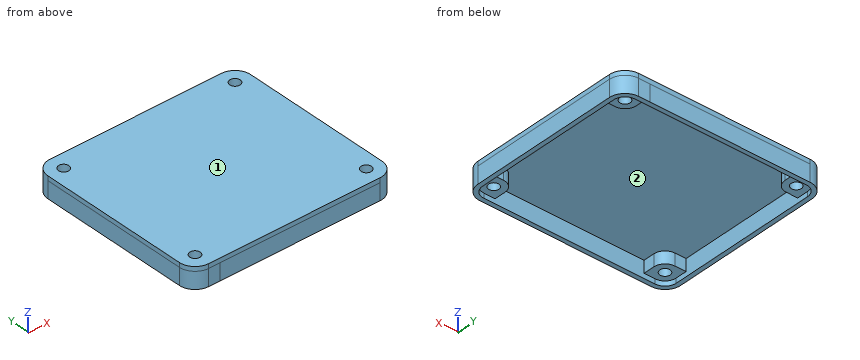
```python
from build123d import *

# Parameters (mm, degrees)
BOSS_EXTRUDE2_START     = -1.618999
SKETCH1_W               = 50.400855702
SKETCH1_H               = 1.5
SKETCH1_W_2             = 1.5
SKETCH1_H_2             = 43.400852302
BOSS_EXTRUDE2_DEPTH     = 5.668998934
SKETCH1_5_R             = 1.74999934
BOSS_EXTRUDE3_DEPTH     = 4.049997769
BOSS_EXTRUDE4_START     = 4.049997821
BOSS_EXTRUDE4_OUTLINE_R = 1.74999934
BOSS_EXTRUDE4_DEPTH     = 1.499999948


# Read off the part's stored shape, not the designer's step: Boss-Extrude4
with BuildPart() as part:
    # Sketch1 → Boss-Extrude2 (new body)
    with BuildSketch(Plane.XY.offset(BOSS_EXTRUDE2_START)):
        with BuildLine():
            Line((7.299572149, 59.8), (3.499574174, 59.8))
            ThreePointArc((3.499574174, 59.8), (-0.247791806, 58.247791067), (-1.8, 54.500424782))
            Line((-1.8, 54.500424782), (-1.8, 50.700426151))
            Line((-1.8, 50.700426151), (-0.3, 50.700426151))
            Line((-0.3, 50.700426151), (-0.3, 54.500425826))
            ThreePointArc((-0.3, 54.500425826), (0.812868735, 57.187131265), (3.499574174, 58.3))
            Line((3.499574174, 58.3), (7.299572149, 58.3))
            Line((7.299572149, 58.3), (7.299572149, 59.8))
        make_face()
        with Locations((32.5, 59.05)):
            Rectangle(SKETCH1_W, SKETCH1_H)
        with BuildLine():
            ThreePointArc((61.500425826, 59.799997355), (65.247788792, 58.247788792), (66.8, 54.500425826))
            Line((66.8, 54.500425826), (66.8, 50.700426151))
            Line((66.8, 50.700426151), (65.3, 50.700426151))
            Line((65.3, 50.700426151), (65.3, 54.500425826))
            ThreePointArc((65.3, 54.500425826), (64.18713049, 57.18713049), (61.500425826, 58.3))
            Line((61.500425826, 58.3), (57.700427851, 58.3))
            Line((57.700427851, 58.3), (57.700427851, 59.8))
            Line((57.700427851, 59.8), (61.500425826, 59.799997355))
        make_face()
        with Locations((66.05, 29)):
            Rectangle(SKETCH1_W_2, SKETCH1_H_2)
        with BuildLine():
            Line((57.700427851, -1.8), (61.500425826, -1.8))
            ThreePointArc((61.500425826, -1.8), (65.247791806, -0.247791067), (66.8, 3.499575218))
            Line((66.8, 3.499575218), (66.8, 7.299573849))
            Line((66.8, 7.299573849), (65.3, 7.299573849))
            Line((65.3, 7.299573849), (65.3, 3.499574174))
            ThreePointArc((65.3, 3.499574174), (64.187131265, 0.812868735), (61.500425826, -0.3))
            Line((61.500425826, -0.3), (57.700427851, -0.3))
            Line((57.700427851, -0.3), (57.700427851, -1.8))
        make_face()
        with Locations((32.5, -1.05)):
            Rectangle(SKETCH1_W, SKETCH1_H)
        with Locations((-1.05, 29)):
            Rectangle(SKETCH1_W_2, SKETCH1_H_2)
        with BuildLine():
            ThreePointArc((3.499576262, -1.800002645), (-0.247793343, -0.24779482), (-1.8, 3.499574174))
            Line((-1.8, 3.499574174), (-1.8, 7.299573849))
            Line((-1.8, 7.299573849), (-0.3, 7.299573849))
            Line((-0.3, 7.299573849), (-0.3, 3.499574174))
            ThreePointArc((-0.3, 3.499574174), (0.812867961, 0.812867961), (3.499574174, -0.3))
            Line((3.499574174, -0.3), (7.299572149, -0.3))
            Line((7.299572149, -0.3), (7.299572149, -1.8))
            Line((7.299572149, -1.8), (3.499576262, -1.800002645))
        make_face()
    extrude(amount=BOSS_EXTRUDE2_DEPTH)

    # Sketch1<5> → Boss-Extrude3 (add)
    # profile 1 of 4: a face of its own
    with BuildSketch(Plane.XY):
        with BuildLine():
            Line((7.299572149, 3.50000232), (7.299572149, -0.3))
            Line((7.299572149, -0.3), (3.499574174, -0.3))
            ThreePointArc((3.499574174, -0.3), (0.812867961, 0.812867961), (-0.3, 3.499574174))
            Line((-0.3, 3.499574174), (-0.3, 7.299573849))
            Line((-0.3, 7.299573849), (3.50000062, 7.299573849))
            ThreePointArc((3.50000062, 7.299573849), (6.186702813, 6.186704015), (7.299572149, 3.50000232))
        make_face()
        with Locations((3.499568884, 3.499568884)):
            Circle(SKETCH1_5_R, mode=Mode.SUBTRACT)
    # profile 2 of 4: a face of its own
    with BuildSketch(Plane.XY):
        with BuildLine():
            Line((7.299572149, 58.3), (3.499574174, 58.3))
            ThreePointArc((3.499574174, 58.3), (0.812868735, 57.187131265), (-0.3, 54.500425826))
            Line((-0.3, 54.500425826), (-0.3, 50.700426151))
            Line((-0.3, 50.700426151), (3.50000062, 50.700426151))
            ThreePointArc((3.50000062, 50.700426151), (6.186703414, 51.813294886), (7.299572149, 54.49999768))
            Line((7.299572149, 54.49999768), (7.299572149, 58.3))
        make_face()
        with Locations((3.499571529, 54.500428471)):
            Circle(SKETCH1_5_R, mode=Mode.SUBTRACT)
    # profile 3 of 4: a face of its own
    with BuildSketch(Plane.XY):
        with BuildLine():
            ThreePointArc((61.500425826, 58.3), (64.18713049, 57.18713049), (65.3, 54.500425826))
            Line((65.3, 54.500425826), (65.3, 50.700426151))
            Line((65.3, 50.700426151), (61.49999938, 50.700426151))
            ThreePointArc((61.49999938, 50.700426151), (58.813296614, 51.813295049), (57.700427851, 54.49999768))
            Line((57.700427851, 54.49999768), (57.700427851, 58.3))
            Line((57.700427851, 58.3), (61.500425826, 58.3))
        make_face()
        with Locations((61.500425826, 54.500425826)):
            Circle(SKETCH1_5_R, mode=Mode.SUBTRACT)
    # profile 4 of 4: a face of its own
    with BuildSketch(Plane.XY):
        with BuildLine():
            Line((57.700427851, -0.3), (61.500425826, -0.3))
            ThreePointArc((61.500425826, -0.3), (64.187131265, 0.812868735), (65.3, 3.499574174))
            Line((65.3, 3.499574174), (65.3, 7.299573849))
            Line((65.3, 7.299573849), (61.49999938, 7.299573849))
            ThreePointArc((61.49999938, 7.299573849), (58.813297215, 6.186703852), (57.700427851, 3.50000232))
            Line((57.700427851, 3.50000232), (57.700427851, -0.3))
        make_face()
        with Locations((61.500428471, 3.499571529)):
            Circle(SKETCH1_5_R, mode=Mode.SUBTRACT)
    extrude(amount=BOSS_EXTRUDE3_DEPTH)

    # Boss-Extrude4 outline → Boss-Extrude4 (add)
    with BuildSketch(Plane.XY.offset(BOSS_EXTRUDE4_START)):
        with BuildLine():
            ThreePointArc((-1.800001322, 3.499574174), (-0.247792408, -0.247793885), (3.499576262, -1.800001322))
            Line((3.499576262, -1.800001322), (61.500425826, -1.8))
            ThreePointArc((61.500425826, -1.8), (65.247791806, -0.247791067), (66.8, 3.499575218))
            Line((66.8, 3.499575218), (66.799998678, 54.500425826))
            ThreePointArc((66.799998678, 54.500425826), (65.247789727, 58.247789727), (61.500425826, 59.799998678))
            Line((61.500425826, 59.799998678), (3.499574174, 59.8))
            ThreePointArc((3.499574174, 59.8), (-0.247791806, 58.247791067), (-1.8, 54.500424782))
            Line((-1.8, 54.500424782), (-1.800001322, 3.499574174))
        make_face()
        with Locations((3.499568884, 3.499568884)):
            Circle(BOSS_EXTRUDE4_OUTLINE_R, mode=Mode.SUBTRACT)
        with Locations((61.500428471, 3.499571529)):
            Circle(BOSS_EXTRUDE4_OUTLINE_R, mode=Mode.SUBTRACT)
        with Locations((3.499571529, 54.500428471)):
            Circle(BOSS_EXTRUDE4_OUTLINE_R, mode=Mode.SUBTRACT)
        with Locations((61.500425826, 54.500425826)):
            Circle(BOSS_EXTRUDE4_OUTLINE_R, mode=Mode.SUBTRACT)
    extrude(amount=BOSS_EXTRUDE4_DEPTH)


solid = part.part
```
CAD build for the part. Positions are in the model's coordinates, mm. Face numbers are marked on the shaded views. Give positions to 0.01 mm unless a question says otherwise; leave off trailing zeros. Use a Markdown table: item, result.
1. Wall check: L1, parallel to Y at x = 52, z = 0.25; L2, parallel to X at y = 12.5, z = -0.5; L3, parallel to Y at x = 4.5, z = 1.5. Give the ranges that are in metal, low to high. Write a range as [from, to].
Check result:
| item | result |
|---|---|
| L1 | y = [-1.8, -0.3], [58.3, 59.8] |
| L2 | x = [-1.8, -0.3], [65.3, 66.8] |
| L3 | y = [-1.8, 2.06], [4.94, 7.17], [50.83, 53.06], [55.94, 59.8] |
2. Slice it at C-C (z = 3.25). Give the number of separate pieces and of enclosed holes in the cut face, plus the area to 3 significant figures.
Check result:
| item | result |
|---|---|
| separate pieces | 1 |
| enclosed holes | 5 |
| area | 538 mm^2 |
3. Mould opens along X. For the marked faces 1 and 2 say: pulls with the +X half, pulls with the -X half, needs draft (parallel to the pull), parting line crosses it, or undercut.
Check result:
| item | result |
|---|---|
| face 1 | needs draft |
| face 2 | undercut |
4. Flat gauge pins, fed straight in: pin 1 (2.5 mm diameter, centred on x = 3.5, y = 2, fed in from -Z); pin 2 (3 mm diameter, centred on y = 1, z = 2.5, fed in from -X); pin 3 (3 mm diameter, centred on y = 1, z = 3, fed in from +X). Where does each tip first touch, or does it go through?
Check result:
| item | result |
|---|---|
| pin 1 | stops at z = 0 |
| pin 2 | stops at x = -1.7 |
| pin 3 | stops at x = 66.7 |
